Autodesk Inventor part; units mm, degrees
ref_plane "YZ Plane" through (0, 0, 0) normal (1, 0, 0) x (0, 1, 0)
ref_plane "XZ Plane" through (0, 0, 0) normal (0, 1, 0) x (-1, 0, 0)
ref_plane "XY Plane" through (0, 0, 0) normal (0, 0, 1) x (1, 0, 0)
sketch "Sketch1" plane through (0, 0, 0) normal (0, 0, 1) x (1, 0, 0)
  line L0 (15, 0) -> (55, 0)
  line L1 (70, 15) -> (70, 15)
  line L2 (55, 30) -> (15, 30)
  line L3 (0, 15) -> (0, 15)
  circle A0 centre (10, 15) radius 5
  circle A1 centre (60, 15) radius 5
  arc A2 (70, 15) -> (55, 30) centre (55, 15) ccw
  arc A3 (55, 0) -> (70, 15) centre (55, 15) ccw
  arc A4 (0, 15) -> (15, 0) centre (15, 15) ccw
  arc A5 (15, 30) -> (0, 15) centre (15, 15) ccw
  point P0 (0, 0)
  point P1 (70, 0)
  point P2 (70, 30)
  point P3 (0, 15)
  dimension "d1" = 30
  dimension "d14" = 10
  dimension "d15" = 10
  dimension "d16" = 10
  dimension "d17" = 50
  dimension "d18" = 15
  dimension "d21" = 15
extrude "Extrusion1" add sketch "Sketch1" along normal blind 3
sketch "Sketch3" plane through (0, 0, 3) normal (0, 0, 1) x (1, 0, 0)
  arc A0 (55, 0) -> (55, 30) centre (55, 15) ccw
  line L0 (55, 30) -> (15, 30)
  arc A1 (15, 30) -> (15, 0) centre (15, 15) ccw
  line L1 (15, 0) -> (55, 0)
  circle A2 centre (60, 15) radius 5
  circle A3 centre (10, 15) radius 5
  line L2 (55, 30) -> (15, 30)
  line L3 (25, 30) -> (25, 0)
  circle A4 centre (10, 15) radius 15
  circle A5 centre (10, 12) radius 15
  point P0 (0, 0)
  point P1 (12.5, 29.7902)
  point P2 (25, 15)
  dimension "d24" = 15
  dimension "d27" = 3
sketch "Sketch4" plane through (0, 0, 3) normal (0, 0, 1) x (1, 0, 0)
  point P0 (0, 0)
extrude "Extrusion3" add sketch "Sketch3" along normal blind 3 contours L1 L3 L0 A0 | L3 A4 A1 L0
sketch "Sketch5" plane through (0, 0, 0) normal (0, 0, -1) x (-1, 0, 0)
  circle A0 centre (-60, 15) radius 5
  circle A1 centre (-10, 15) radius 5
  circle A2 centre (-40, 15) radius 2.5
  line L0 (-25, 0) -> (-25, 15)
  point P0 (0, 0)
  dimension "d30" = 5
  dimension "d33" = 35
  dimension "d34" = 10
  dimension "d36" = 15
extrude "Extrusion4" cut sketch "Sketch5" against normal blind 0.1 contours A2
sketch "Sketch6" plane through (0, 0, 6) normal (0, 0, 1) x (1, 0, 0)
  circle A0 centre (40, 15) radius 2.5
  point P0 (0, 0)
extrude "Extrusion5" cut sketch "Sketch6" against normal blind 0.1
equation "\"d14\" = d6"
equation "\"d15\" = d14"
equation "\"d16\" = d15"
equation "\"d18\" = 0.5 * d1"
equation "\"d21\" = 0.5 * d1"
equation "\"d19\" = d11"
equation "\"d24\" = 0.5 * d0"
equation "\"d27\" = 0.1 * d0"
equation "\"d25\" = d11"
equation "\"d36\" = 0.5 * d33 - 0.25 * d34"
properties part number "GripP3"
Work out the finished part from the listing and answer in its coordinate system (mm). A direction names the side the tool comes from. Give positions to 0.01 mm unless a question says otherwise; leave off trailing zeros. Order: outer loops, then holes, each group sorted by start corner. A loop starts at its lowest first (then second) coordinate and runs counter-clockwise, first axis right, second up.
1. Section B-B, the plane z = 4.6 is taken. Determine the outline of the cut face in (x, y).
Result sheet:
outline: (12.5, 29.79) arc R15 cw to (25, 15) - (25, 0) - (55, 0) arc R15 ccw to (55, 30) - (15, 30) arc R15 ccw to start; hole circle Ø10 at (60, 15)
2. For faces 1 (the flat face through (15, 12, 3)), 2 (the flat face through (40, 15, 0.1)), 3 (the flat face through (35, 0, 3)), determine the directions among +Z, -Z, +X, -X, +Y, -Y from which every point of the face is accessible in a straight line to the end or side of a thin tool.
Result sheet:
face 1: +Z, -X, -Y
face 2: -Z
face 3: +Z, -Z, +X, -X, -Y
3. Straight lines are drawn through the part: L1, parallel to Y at x = 40, z = 0.05; L2, parallel to X at y = 14.5, z = 1.95; L3, parallel to X at y = 18, z = 3.2. For each, find the intervals that lie inside material, in ascending order.
Result sheet:
L1: y = 0 to 12.5, 17.5 to 30
L2: x = 0.01 to 5.03, 14.97 to 55.03, 64.97 to 69.99
L3: x = 24.7 to 56, 64 to 69.7
4. Section A-A, the plane x = 60 is taken. Determine the outline of the cut face in (y, z), and give its area (3 significant figures).
Result sheet:
outline: (0.86, 0) - (10, 0) - (10, 6) - (0.86, 6) - close; (20, 0) - (29.14, 0) - (29.14, 6) - (20, 6) - close
area: 110 mm2
5. Section C-C, the plane x = 10 is taken. Determine the outline of the cut face in (y, z), and give its area (3 significant figures).
Result sheet:
outline: (0.86, 0) - (10, 0) - (10, 3) - (0.86, 3) - close; (20, 0) - (29.14, 0) - (29.14, 3) - (20, 3) - close
area: 54.9 mm2
6. Section D-D, the plane y = 21.5 is taken. Determine the outline of the cut face in (x, z).
Result sheet:
outline: (1.48, 0) - (68.52, 0) - (68.52, 6) - (23.52, 6) - (23.52, 3) - (1.48, 3) - close
7. Each of these flat-tipped pins is pushed along its axis until it touches: P1, Ø1.5, axis at y = 3.5, z = 2.5, coming from the +X side; P2, Ø12.5, axis at x = 15, y = 22, coming from the +Z side; P3, Ø2.5, axis at x = 40, y = 14.5, coming from the -Z side. Where does it stop, or does it pass through?
Result sheet:
P1: stops at x = 65.46
P2: stops at z = 3
P3: stops at z = 0.1
8. The mould has two halves that part along X. Classify faces 4 (the cylindrical face through (56, 18, 3)), 5 (the cylindrical face through (21.361, 24.795, 4.479)), 6 (the flat face through (40, 15, 5.9)), 7 (the cylindrical face through (70, 15, 3)): released by +X, released by -X, zero draft, split by the parting line, or undercut.
Result sheet:
face 4: undercut
face 5: released by -X
face 6: undercut
face 7: released by +X
